Drawing for the job (mm, zero at the part's lowest x, y, z). Coordinates: 2 decimals unless noted, no trailing zeros. Loops run counter-clockwise (first coordinate to the right, second up) from the corner with the lowest first, then second, coordinate; pieces in that order, holes last. Notation, with made-up numbers: (33.5, -3.5) -> (90.5, -3.5) arc R19 ccw to (90.5, 25.5) -> close; hole circle Ø3 at (-34, 74.5). An arc over 180 degrees is marked (long way). Write each question's results on one line, items separated by ' | '.
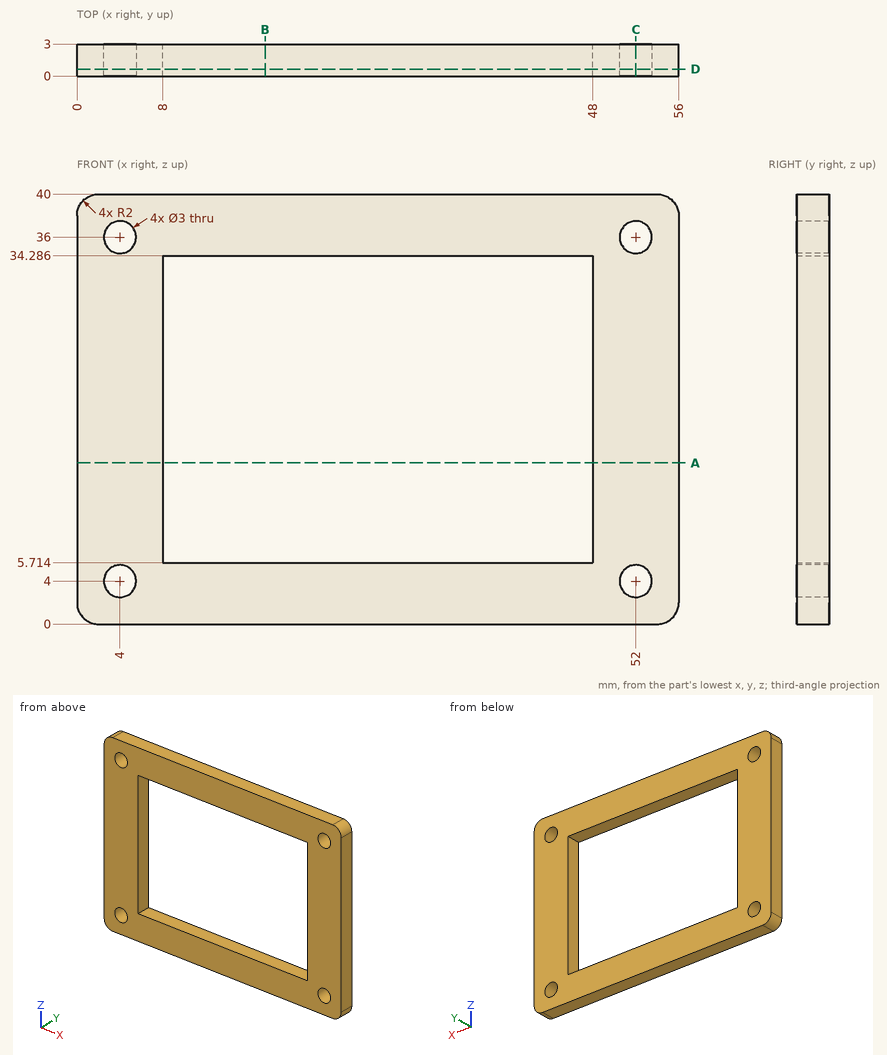
1) Slice it at C-C (x = 52). Write the cut outline in (y, z), then the cut area to 3 significant figures.
Outcome:
outline: (0, 0) -> (3, 0) -> (3, 2.5) -> (0, 2.5) -> close; (0, 5.5) -> (3, 5.5) -> (3, 34.5) -> (0, 34.5) -> close; (0, 37.5) -> (3, 37.5) -> (3, 40) -> (0, 40) -> close | area: 102 mm^2
2) Slice it at B-B (x = 17.5). Write the cut outline in (y, z), then the cut area to 3 significant figures.
Outcome:
outline: (0, 0) -> (3, 0) -> (3, 5.71) -> (0, 5.71) -> close; (0, 34.29) -> (3, 34.29) -> (3, 40) -> (0, 40) -> close | area: 34.3 mm^2
3) Drill centre lines: L1, parallel to X at y = 1.7, z = 4; L2, parallel to Z at x = 4, y = 1.8; L3, parallel to Z at x = 23, y = 2.65. Where is each one in solid material? Low to high. Write a range as from..to.
Outcome:
L1: x = 0..2.5, 5.5..50.5, 53.5..56 | L2: z = 0..2.5, 5.5..34.5, 37.5..40 | L3: z = 0..5.71, 34.29..40
4) Slice it at A-A (z = 15). Write the cut outline in (x, y).
Outcome:
outline: (0, 0) -> (8, 0) -> (8, 3) -> (0, 3) -> close; (48, 0) -> (56, 0) -> (56, 3) -> (48, 3) -> close
5) Pin check, flat tip, straight feed: pin 1 (1.8 mm diameter, centred on x = 52, z = 36, fed in from -Y). Stop position of the tip, or through.
Outcome:
pin 1: passes through
6) Slice it at D-D (y = 0.65). Write the cut outline in (x, z), then the cut area to 3 significant figures.
Outcome:
outline: (0, 2) arc R2 ccw to (2, 0) -> (54, 0) arc R2 ccw to (56, 2) -> (56, 38) arc R2 ccw to (54, 40) -> (2, 40) arc R2 ccw to (0, 38) -> close; hole circle Ø3 at (4, 4); hole circle Ø3 at (4, 36); hole (8, 5.71) -> (48, 5.71) -> (48, 34.29) -> (8, 34.29) -> close; hole circle Ø3 at (52, 4); hole circle Ø3 at (52, 36) | area: 1,070 mm^2
